from build123d import *

# Parameters (mm, degrees)
ESQUISSE1_R                  = 35
ESQUISSE1_R_2                = 32
BOSS_EXTRU_1_DEPTH           = 70
BOSS_EXTRU_2_DEPTH           = 70
ESQUISSE3_R                  = 3.2
ENL_V_MAT_EXTRU_1_DEPTH      = 20
ENL_V_MAT_EXTRU_1_DEPTH_BACK = 20
ESQUISSE5_W                  = 100
ESQUISSE5_H                  = 50
ENL_V_MAT_EXTRU_3_DEPTH      = 71
ESQUISSE7_W                  = 10
ESQUISSE7_H                  = 70
ESQUISSE7_R                  = 3.2
BOSS_EXTRU_3_DEPTH           = 8
BOSS_EXTRU_5_DEPTH           = 70
ESQUISSE10_R                 = 32
ENL_V_MAT_EXTRU_4_DEPTH      = 20
CONG_2_R                     = 2
BOSS_EXTRU_6_START           = -1.5
ESQUISSE11_R                 = 3.2
BOSS_EXTRU_6_DEPTH           = 33


with BuildPart() as part:
    # Esquisse1 → Boss.-Extru.1 (new body)
    with BuildSketch(Plane.XY):
        Circle(ESQUISSE1_R)
        Circle(ESQUISSE1_R_2, mode=Mode.SUBTRACT)
    extrude(amount=BOSS_EXTRU_1_DEPTH)

    # Esquisse2 → Boss.-Extru.2 (add)
    with BuildSketch(Plane.XY.offset(70)):
        with BuildLine():
            Line((-7.5, 31.108680461), (-7.5, -31.108680461))
            ThreePointArc((-7.5, -31.108680461), (-12.685066047, -29.378378093), (-17.5, -26.790856649))
            Line((-17.5, -26.790856649), (-17.5, 26.790856649))
            ThreePointArc((-17.5, 26.790856649), (-12.685066047, 29.378378093), (-7.5, 31.108680461))
        make_face()
        with BuildLine():
            Line((17.5, -26.790856649), (17.5, 26.790856649))
            ThreePointArc((17.5, 26.790856649), (12.685066047, 29.378378093), (7.5, 31.108680461))
            Line((7.5, 31.108680461), (7.5, -31.108680461))
            ThreePointArc((7.5, -31.108680461), (12.685066047, -29.378378093), (17.5, -26.790856649))
        make_face()
    extrude(amount=-BOSS_EXTRU_2_DEPTH)

    # Esquisse3 → Enlèv. mat.-Extru.1 (cut, two sides)
    with BuildSketch(Plane(origin=(0, 0, 0), x_dir=(1, 0, 0), z_dir=(0, 1, 0))) as enl_v_mat_extru_1_sk:
        with Locations((-12.5, -10)):
            Circle(ESQUISSE3_R)
        with Locations((-12.5, -40)):
            Circle(ESQUISSE3_R)
        with Locations((12.5, -40)):
            Circle(ESQUISSE3_R)
        with Locations((12.5, -10)):
            Circle(ESQUISSE3_R)
    extrude(amount=ENL_V_MAT_EXTRU_1_DEPTH, mode=Mode.SUBTRACT)
    extrude(enl_v_mat_extru_1_sk.sketch, amount=-ENL_V_MAT_EXTRU_1_DEPTH_BACK, mode=Mode.SUBTRACT)

    # Esquisse5 → Enlèv. mat.-Extru.3 (cut, through all)
    with BuildSketch(Plane.XY.offset(70)):
        with Locations((0, -31.5)):
            Rectangle(ESQUISSE5_W, ESQUISSE5_H)
    extrude(amount=-ENL_V_MAT_EXTRU_3_DEPTH, mode=Mode.SUBTRACT)

    # Esquisse7 → Boss.-Extru.3 (add)
    with BuildSketch(Plane.XZ.offset(6.5)):
        with Locations((-12.5, 35)):
            Rectangle(ESQUISSE7_W, ESQUISSE7_H)
        with Locations((-12.5, 40)):
            Circle(ESQUISSE7_R, mode=Mode.SUBTRACT)
        with Locations((-12.5, 10)):
            Circle(ESQUISSE7_R, mode=Mode.SUBTRACT)
        with Locations((12.5, 35)):
            Rectangle(ESQUISSE7_W, ESQUISSE7_H)
        with Locations((12.5, 40)):
            Circle(ESQUISSE7_R, mode=Mode.SUBTRACT)
        with Locations((12.5, 10)):
            Circle(ESQUISSE7_R, mode=Mode.SUBTRACT)
    extrude(amount=BOSS_EXTRU_3_DEPTH)

    # Esquisse8 → Boss.-Extru.5 (add)
    with BuildSketch(Plane.XY.offset(70)):
        with BuildLine():
            Line((32.889241728, -11.970705016), (30.070163865, -10.944644586))
            ThreePointArc((30.070163865, -10.944644586), (30.781853005, -8.745142969), (31.332890068, -6.5))
            Line((31.332890068, -6.5), (34.391132578, -6.5))
            ThreePointArc((34.391132578, -6.5), (33.751212497, -9.265832665), (32.889241728, -11.970705016))
        make_face()
        with BuildLine():
            Line((-32.889241728, -11.970705016), (-30.070163865, -10.944644586))
            ThreePointArc((-30.070163865, -10.944644586), (-30.781853005, -8.745142969), (-31.332890068, -6.5))
            Line((-31.332890068, -6.5), (-34.391132578, -6.5))
            ThreePointArc((-34.391132578, -6.5), (-33.751212497, -9.265832665), (-32.889241728, -11.970705016))
        make_face()
    extrude(amount=-BOSS_EXTRU_5_DEPTH)

    # Esquisse10 → Enlèv. mat.-Extru.4 (cut)
    with BuildSketch(Plane.XY.offset(70)):
        Circle(ESQUISSE10_R)
    extrude(amount=-ENL_V_MAT_EXTRU_4_DEPTH, mode=Mode.SUBTRACT)

    # Congé2
    cong_2_edges = [part.edges().sort_by_distance(p)[0] for p in [
        (-17.5, 26.790856649, 25),
        (-7.5, 31.108680461, 25),
        (7.5, 31.108680461, 25),
        (17.5, 26.790856649, 25),
    ]]
    fillet(cong_2_edges, radius=CONG_2_R)

    # Esquisse11 → Boss.-Extru.6 (add)
    with BuildSketch(Plane.XZ.offset(14.5).offset(BOSS_EXTRU_6_START)):
        with Locations((12.5, 10)):
            Circle(ESQUISSE11_R)
        with Locations((12.5, 40)):
            Circle(ESQUISSE11_R)
        with Locations((-12.5, 40)):
            Circle(ESQUISSE11_R)
        with Locations((-12.5, 10)):
            Circle(ESQUISSE11_R)
    extrude(amount=-BOSS_EXTRU_6_DEPTH)


solid = part.part
Part model, mm, in its own coordinate system. A direction names the side the tool comes from. Give positions to 0.01 mm unless a question says otherwise; leave off trailing zeros. Loops run counter-clockwise (first coordinate to the right, second up) from the corner with the lowest first, then second, coordinate; pieces in that order, holes last. Notation, with made-up numbers: (-8, 79) -> (39, 79) arc R19 cw to (39, 89) -> close; hole circle Ø5 at (-25.75, 74). An arc over 180 degrees is marked (long way). Write each question's results on one line, items separated by ' | '. Start each with the question number.
Q1. Band-saw the part on C-C on y = 20. List the corners of the cut face in (x, z).
Q2. Which spindle directions (+Z, -Z, +X, -X, +Y, -Y) get a long thin tool onto all of the face, cutting with end or side? Do faces 4 (the face through (12.083, -13.74, 43.173)), 5 (the face through (-31.499, -11.465, 35.49)), 6 (the face through (12, -14.5, 25)). Say none if no direction does.
Q3. Pin check, flat tips, straight feed: P1, Ø1.5, axis at y = 8, z = 9, coming from the -X side; P2, Ø5, axis at x = -13, z = 9, coming from the -Y side; P3, Ø12, axis at x = -15.5, y = 7, coming from the +Z side; P4, Ø8, axis at x = -12.5, z = 58.5, coming from the -Y side. Stop position of each tip, or through.
Q4. Wall check: L1, parallel to Z at x = -12.5, y = -13.9; L2, parallel to X at y = 0, z = 42; L3, parallel to X at y = -1, z = 54.5. Give the ranges that are in metal, low to high.
Q5. Band-saw the part on B-B on z = 53. List the corners of the cut face in (x, y).
Q6. Band-saw the part on D-D on x = -12.5. List the corners of the cut face in (y, z).
Q7. Pull direction X, two halves, no side cores. Call faces 1 (the face through (0, 33, 70)), 2 (the face through (12, -13, 10)), 3 (the face through (18.692, 24.628, 24.65)): +X half, -X half, draft (parallel to the pull), parting line (faces both ways), or undercut.
Q8. Band-saw the part on A-A on y = 0. List the corners of the cut face in (x, z), plus the area to 3 significant figures.
Results are:
1) outline: (-28.72, 0) -> (-24.98, 0) -> (-24.98, 70) -> (-28.72, 70) -> close; (-17.5, 0) -> (-7.5, 0) -> (-7.5, 50) -> (-17.5, 50) -> close; (7.5, 0) -> (17.5, 0) -> (17.5, 50) -> (7.5, 50) -> close; (24.98, 0) -> (28.72, 0) -> (28.72, 70) -> (24.98, 70) -> close
2) face 4: -Y | face 5: +Z, -Z, -Y | face 6: +Z, -Z, +X, -X, -Y
3) P1: stops at x = -34.24 | P2: stops at y = -14.5 | P3: stops at z = 50 | P4: stops at y = 27.42
4) L1: z = 0 to 6.8, 13.2 to 36.8, 43.2 to 50 | L2: x = -35 to -32, -17.5 to -7.5, 7.5 to 17.5, 32 to 35 | L3: x = -34.99 to -31.98, 31.98 to 34.99
5) outline: (-32.89, -11.97) -> (-30.07, -10.94) arc R32 cw (long way) to (30.07, -10.94) -> (32.89, -11.97) arc R35 ccw (long way) to start
6) outline: (-14.5, 0) -> (32.69, 0) -> (32.69, 70) -> (29.46, 70) -> (29.46, 50) -> (-14.5, 50) -> (-14.5, 43.2) -> (-13, 43.2) -> (-13, 36.8) -> (-14.5, 36.8) -> (-14.5, 13.2) -> (-13, 13.2) -> (-13, 6.8) -> (-14.5, 6.8) -> close
7) face 1: draft | face 2: undercut | face 3: undercut
8) outline: (-35, 0) -> (-32, 0) -> (-32, 70) -> (-35, 70) -> close; (-17.5, 0) -> (-7.5, 0) -> (-7.5, 50) -> (-17.5, 50) -> close; (7.5, 0) -> (17.5, 0) -> (17.5, 50) -> (7.5, 50) -> close; (32, 0) -> (35, 0) -> (35, 70) -> (32, 70) -> close | area: 1,420 mm²
